The model under review builds one solid part; all positions refer to its coordinate system, in mm. Give positions to 0.01 mm unless a question says otherwise; leave off trailing zeros. Order: outer loops, then holes, each group sorted by start corner. A loop starts at its lowest first (then second) coordinate and runs counter-clockwise, first axis right, second up.
```python
from build123d import *

# Parameters (mm, degrees)
SKETCH2_R               = 1
BOSS_EXTRUDE1_DEPTH     = 7.5
SKETCH4_OUTSIDE_W       = 5.604
SKETCH4_OUTSIDE_H       = 5.604
SKETCH4_OUTSIDE_R       = 0.8
CUT_EXTRUDE1_DEPTH      = 1.5
CUT_EXTRUDE1_DEPTH_BACK = 1.5
SKETCH5_R               = 0.6
CUT_EXTRUDE2_DEPTH      = 7.5


with BuildPart() as part:
    # Sketch2 → Boss-Extrude1 (new body)
    with BuildSketch(Plane(origin=(0, 0, 0), x_dir=(1, 0, 0), z_dir=(0, 1, 0))):
        Circle(SKETCH2_R)
    extrude(amount=BOSS_EXTRUDE1_DEPTH)

    # Sketch4 outside → Cut-Extrude1 (cut, two sides)
    with BuildSketch(Plane(origin=(0, 3.75, 0), x_dir=(1, 0, 0), z_dir=(0, 1, 0))) as cut_extrude1_sk:
        Rectangle(SKETCH4_OUTSIDE_W, SKETCH4_OUTSIDE_H)
        Circle(SKETCH4_OUTSIDE_R, mode=Mode.SUBTRACT)
    extrude(amount=CUT_EXTRUDE1_DEPTH, mode=Mode.SUBTRACT)
    extrude(cut_extrude1_sk.sketch, amount=-CUT_EXTRUDE1_DEPTH_BACK, mode=Mode.SUBTRACT)

    # Sketch5 → Cut-Extrude2 (cut)
    with BuildSketch(Plane(origin=(0, 7.5, 0), x_dir=(1, 0, 0), z_dir=(0, 1, 0))):
        Circle(SKETCH5_R)
    extrude(amount=-CUT_EXTRUDE2_DEPTH, mode=Mode.SUBTRACT)


solid = part.part
```
1. Take a section at A-A (x = 0). Write out the cut boundary in (y, z), and give its area (3 significant figures).
2. Take a section at B-B (z = 0). Write out the cut boundary in (x, y).
3. Insertion check: pin 1 (1 mm diameter, centred on x = 0, z = 0, fed in from +Y); pin 2 (1 mm diameter, centred on y = 3.5, z = 0.5, fed in from -X). Each pin has a flat end and moves straight along its axis. Give the tip position at first contact, or say it passes through.
4. To check wall thickness, follow line 1 (Z direction, x = 0, y = 2.75); line 2 (Z direction, x = 0, y = 6.25). State the ranges of each line that lie inside material, in increasing order.
5. Take a section at C-C (y = 1.5). Write out the cut boundary in (x, z).
6. Draft analysis for pull direction Y (two halves, no side actions). For faces 1 (the cylindrical face through (-0.63, 3.77, 0.49)), 2 (the cylindrical face through (0, 6, 1)), state which applies: pulls with the +Y half, pulls with the -Y half, needs draft (parallel to the pull), parting line crosses it, or undercut.
7. Take a section at D-D (x = -0.7). Write out the cut boundary in (y, z), and give its area (3 significant figures).
Answer:
1. outline: (0, -1) - (2.25, -1) - (2.25, -0.8) - (5.25, -0.8) - (5.25, -1) - (7.5, -1) - (7.5, -0.6) - (0, -0.6) - close; (0, 0.6) - (7.5, 0.6) - (7.5, 1) - (5.25, 1) - (5.25, 0.8) - (2.25, 0.8) - (2.25, 1) - (0, 1) - close
1. area: 4.80 mm2
2. outline: (-1, 0) - (-0.6, 0) - (-0.6, 7.5) - (-1, 7.5) - (-1, 5.25) - (-0.8, 5.25) - (-0.8, 2.25) - (-1, 2.25) - close; (0.6, 0) - (1, 0) - (1, 2.25) - (0.8, 2.25) - (0.8, 5.25) - (1, 5.25) - (1, 7.5) - (0.6, 7.5) - close
3. pin 1: passes through
3. pin 2: stops at x = -0.8
4. line 1: z = -0.8 to -0.6, 0.6 to 0.8
4. line 2: z = -1 to -0.6, 0.6 to 1
5. outline: circle Ø2 at (0, 0); hole circle Ø1.2 at (0, 0)
6. face 1: undercut
6. face 2: needs draft
7. outline: (0, -0.71) - (2.25, -0.71) - (2.25, -0.39) - (5.25, -0.39) - (5.25, -0.71) - (7.5, -0.71) - (7.5, 0.71) - (5.25, 0.71) - (5.25, 0.39) - (2.25, 0.39) - (2.25, 0.71) - (0, 0.71) - close
7. area: 8.75 mm2
